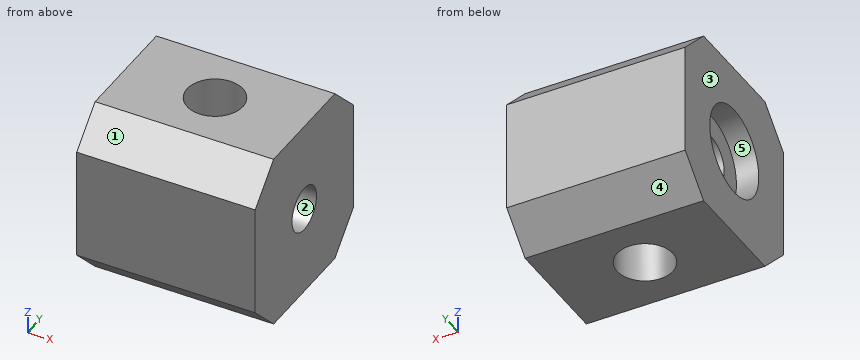
Autodesk Inventor part; units mm, degrees
ref_plane "YZ Plane" through (0, 0, 0) normal (1, 0, 0) x (0, 1, 0)
ref_plane "XZ Plane" through (0, 0, 0) normal (0, 1, 0) x (-1, 0, 0)
ref_plane "XY Plane" through (0, 0, 0) normal (0, 0, 1) x (1, 0, 0)
sketch "Skizze2" plane through (0, 0, 0) normal (1, 0, 0) x (0, 1, 0)
  line L0 (4, 4) -> (-4, 4)
  line L1 (-4, 4) -> (-4, -4)
  line L2 (-4, -4) -> (4, -4)
  line L3 (4, -4) -> (4, 4)
  point P0 (0, 0)
  point P1 (0, 0)
  dimension "d7" = 8
  dimension "d8" = 8
  dimension "d9" = 4
  dimension "d10" = 4
extrude "Extrusion1" add sketch "Skizze2" along normal blind 8
chamfer "Fase1" distance 1.5 angle 45 4 edges at (4, 4, 4) (4, 4, -4) (4, -4, 4) (4, -4, -4)
hole "Bohrung1" at (0, 0, 0) direction (1, 0, 0) diameter 2 end through all counterbore diameter 4 counterbore depth 1
sketch "Skizze3" plane through (0, -2.5, -4) normal (0, 0, -1) x (-1, 0, 0)
  line L0 (0, 0) -> (0, 5)
  line L1 (-8, -1.5) -> (0, -1.5)
  point P0 (0, 2.5)
  point P1 (-4, 2.5)
  dimension "d23" = 4
  dimension "d24" = 4
hole "Bohrung2" at (4, 0, -4) direction (0, 0, 1) diameter 2.5 end through all
thread "Gewinde1"
properties part number "Aluminium_Block_Motor"
Check sheet for the modelled part. Datum: model origin and axes. Units: mm. Face numbers are marked on the shaded views. A direction names the side the tool comes from. Round coordinates to 2 decimals unless told otherwise and drop trailing zeros. Order: outer loops, then holes, each group sorted by start corner. A loop starts at its lowest first (then second) coordinate and runs counter-clockwise, first axis right, second up.
(1) Cross-section at C-C, the plane y = 0. Enter the section's corners in (x, z).
(2) Access from +Z, -Z, +X, -X, +Y, -Y to the whole of each face (thin tool, end or side, straight path). Record for the marked faces 4 and 5.
(3) Draft check along Z on the marked faces 1, 2 and 3. Enter one of: pulls with the +Z half, pulls with the -Z half, needs draft (parallel to the pull), parting line crosses it, or undercut.
(4) Cross-section at D-D, the plane x = 2.5. Enter the section's corners in (y, z), and give its area (3 significant figures).
(5) Cross-section at A-A, the plane z = 0. Enter the section's corners in (x, y), and give its area (3 significant figures).
(6) Go/stop test with a flat-tipped pin: P1, Ø3, axis at y = 0, z = 0, coming from the -X side. Record where the tip stops, or that it passes through.
(7) Cross-section at B-B, the plane x = 4. Enter the section's corners in (y, z), and give its area (3 significant figures).
(8) Scan lines: probe 1 along X at (y, z) = (1, -3.25); probe 2 along Y at (x, z) = (6.2, 0). Record each from-to range of solid material in increasing order.
Check sheet entries:
1. outline: (0, -4) - (2.75, -4) - (2.75, -1) - (1, -1) - (1, -2) - (0, -2) - close; (0, 2) - (1, 2) - (1, 1) - (2.75, 1) - (2.75, 4) - (0, 4) - close; (5.25, -4) - (8, -4) - (8, -1) - (5.25, -1) - close; (5.25, 1) - (8, 1) - (8, 4) - (5.25, 4) - close
2. face 4: -Z, +X, -X, +Y
2. face 5: -X
3. face 1: pulls with the +Z half
3. face 2: undercut
3. face 3: needs draft
4. outline: (-4, -2.5) - (-2.5, -4) - (2.5, -4) - (4, -2.5) - (4, 2.5) - (2.5, 4) - (-2.5, 4) - (-4, 2.5) - close; hole circle Ø2 at (0, 0)
4. area: 56.4 mm2
5. outline: (0, -4) - (8, -4) - (8, -1) - (4.75, -1) arc R1.25 cw to (3.25, -1) - (1, -1) - (1, -2) - (0, -2) - close; (0, 2) - (1, 2) - (1, 1) - (3.25, 1) arc R1.25 cw to (4.75, 1) - (8, 1) - (8, 4) - (0, 4) - close
5. area: 45.5 mm2
6. P1: stops at x = 1
7. outline: (-4, -2.5) - (-2.5, -4) - (-1.25, -4) - (-1.25, 4) - (-2.5, 4) - (-4, 2.5) - close; (1.25, -4) - (2.5, -4) - (4, -2.5) - (4, 2.5) - (2.5, 4) - (1.25, 4) - close
7. area: 39.5 mm2
8. probe 1: x = 0 to 3.25, 4.75 to 8
8. probe 2: y = -4 to -1, 1 to 4
